Geometry: final body of the model. Coordinates: model frame, mm. Face numbers are marked on the shaded views. A direction names the side the tool comes from. Round coordinates to 2 decimals unless told otherwise and drop trailing zeros. Loops run counter-clockwise (first coordinate to the right, second up) from the corner with the lowest first, then second, coordinate; pieces in that order, holes last. Notation, with made-up numbers: (-4.75, -35) -> (50.25, -35) arc R36 cw to (50.25, 4) -> close; hole circle Ø5 at (-14.75, -34.5). An arc over 180 degrees is marked (long way). Answer in a Markdown table with one row per item.
```python
from build123d import *

# Parameters (mm, degrees)
SKETCH_W        = 83
SKETCH_H        = 20
PAD_DEPTH       = 3
SKETCH001_W     = 3
SKETCH001_H     = 20
PAD001_DEPTH    = 25
SKETCH002_W     = 30
SKETCH002_H     = 20
PAD002_DEPTH    = 50
POCKET_DEPTH    = 20.001
POCKET001_DEPTH = 53.001
SKETCH006_W     = 3
SKETCH006_H     = 20
PAD003_DEPTH    = 10
SKETCH007_W     = 20
SKETCH007_H     = 3
PAD004_DEPTH    = 5


with BuildPart() as part:
    # Sketch → Pad (new body)
    with BuildSketch(Plane.XY):
        Rectangle(SKETCH_W, SKETCH_H)
    extrude(amount=PAD_DEPTH)

    # Sketch001 → Pad001 (new body)
    with BuildSketch(Plane.XY.offset(3)):
        with Locations((-40, 0)):
            Rectangle(SKETCH001_W, SKETCH001_H)
    extrude(amount=PAD001_DEPTH)

    # Sketch002 → Pad002 (new body)
    with BuildSketch(Plane.XY.offset(3)):
        with Locations((14.5, 0)):
            Rectangle(SKETCH002_W, SKETCH002_H)
    extrude(amount=PAD002_DEPTH)

    # Sketch004 → Pocket (cut, through all)
    with BuildSketch(Plane.XZ.offset(10)):
        with BuildLine():
            Line((2.5, 53), (6.936769, 23.329896))
            ThreePointArc((6.936769, 23.329896), (11.333368, 13.220729), (20.195517, 6.664232))
            Line((20.195517, 6.664232), (29.5, 3))
            Line((63.265705, 66.309877), (29.5, 3))
            Line((2.5, 53), (63.265705, 66.309877))
        make_face()
    extrude(amount=-POCKET_DEPTH, mode=Mode.SUBTRACT)

    # Sketch005 → Pocket001 (cut, through all)
    with BuildSketch(Plane(origin=(0, 0, 0), x_dir=(1, 0, 0), z_dir=(0, 0, -1))):
        with BuildLine():
            ThreePointArc((-25.5, 7), (-32.5, 0), (-25.5, -7))
            Line((-25.5, -7), (29.5, -7))
            ThreePointArc((29.5, -7), (36.5, 0), (29.5, 7))
            Line((-25.5, 7), (29.5, 7))
        make_face()
    extrude(amount=-POCKET001_DEPTH, mode=Mode.SUBTRACT)

    # Sketch006 → Pad003 (new body)
    with BuildSketch(Plane(origin=(0, 0, 0), x_dir=(1, 0, 0), z_dir=(0, 0, -1))):
        with Locations((40, 0)):
            Rectangle(SKETCH006_W, SKETCH006_H)
    extrude(amount=PAD003_DEPTH)

    # Sketch007 → Pad004 (new body)
    with BuildSketch(Plane(origin=(38.5, 0, 0), x_dir=(0, -1, 0), z_dir=(-1, 0, 0))):
        with Locations((0, -8.5)):
            Rectangle(SKETCH007_W, SKETCH007_H)
    extrude(amount=PAD004_DEPTH)


solid = part.part
```
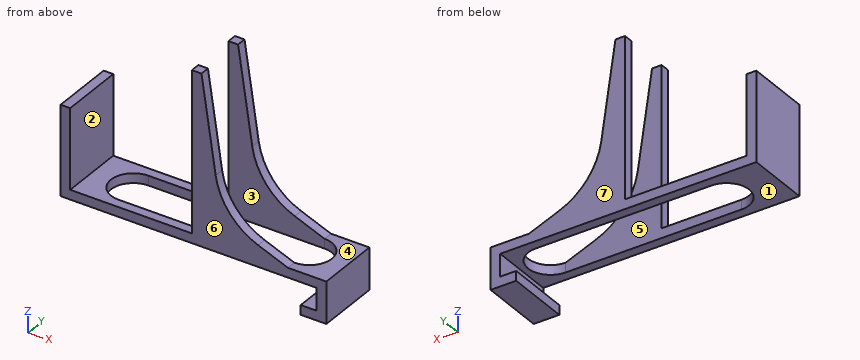
Item 1: Cut plane D-D (z = -5). Output: boundary loops of the cut face in (x, y), then the cut area to 3 significant figures.
Answer:
| item | result |
|---|---|
| outline | (38.5, -10) -> (41.5, -10) -> (41.5, 10) -> (38.5, 10) -> close |
| area | 60.0 mm² |
Item 2: Pin query (flat end, axial travel): pin 1 Ø12 at (x, y) = (19.5, -7) entering from +Z; pin 2 Ø3.5 at (x, y) = (-40.5, -4.5) entering from +Z; pin 3 Ø6 at (y, z) = (-1.5, 18.5) entering from +X. Return the tip coordinate at first contact, or that it passes through.
Answer:
| item | result |
|---|---|
| pin 1 | stops at z = 10.88 |
| pin 2 | stops at z = 28 |
| pin 3 | stops at x = -38.5 |
Item 3: Cut plane A-A (x = -23.5). Output: boundary loops of the cut face in (y, z), then the cut area to 3 significant figures.
Answer:
| item | result |
|---|---|
| outline | (-10, 0) -> (-7, 0) -> (-7, 3) -> (-10, 3) -> close; (7, 0) -> (10, 0) -> (10, 3) -> (7, 3) -> close |
| area | 18.0 mm² |
Item 4: Reachability of the marked faces 1, 2 and 3 from +Z, -Z, +X, -X, +Y, -Y: full face, straight path, thin tool, end or side. Return the list, or none.
Answer:
| item | result |
|---|---|
| face 1 | -X, +Y, -Y |
| face 2 | +Z, +Y, -Y |
| face 3 | +Z, -Z |
Item 5: Draft query along Y for the marked faces 4, 5, 6 and 7. Return one class per face: pulls with the +Y half, pulls with the -Y half, needs draft (parallel to the pull), parting line crosses it, or undercut.
Answer:
| item | result |
|---|---|
| face 4 | needs draft |
| face 5 | undercut |
| face 6 | pulls with the -Y half |
| face 7 | pulls with the +Y half |
Item 6: Cut plane B-B (y = -5.75). Output: boundary loops of the cut face in (x, z), then the cut area to 3 significant figures.
Answer:
| item | result |
|---|---|
| outline | (-41.5, 0) -> (-29.49, 0) -> (-29.49, 3) -> (-38.5, 3) -> (-38.5, 28) -> (-41.5, 28) -> close; (33.49, 0) -> (38.5, 0) -> (38.5, -7) -> (33.5, -7) -> (33.5, -10) -> (41.5, -10) -> (41.5, 3) -> (33.49, 3) -> close |
| area | 180 mm² |
Item 7: Cut plane C-C (y = 8.25). Output: boundary loops of the cut face in (x, z), then the cut area to 3 significant figures.
Answer:
| item | result |
|---|---|
| outline | (-41.5, 0) -> (38.5, 0) -> (38.5, -7) -> (33.5, -7) -> (33.5, -10) -> (41.5, -10) -> (41.5, 3) -> (29.5, 3) -> (20.2, 6.66) arc R21.3 cw to (6.94, 23.33) -> (2.5, 53) -> (-0.5, 53) -> (-0.5, 3) -> (-38.5, 3) -> (-38.5, 28) -> (-41.5, 28) -> close |
| area | 810 mm² |
Item 8: Line query: probe 1 along Y at (x, z) = (2, 36.5); probe 2 along Z at (x, y) = (34, 3.75); probe 3 along X at (y, z) = (4, 14.5). Output: solid intervals per line, ascending. Write a range as [from, to].
Answer:
| item | result |
|---|---|
| probe 1 | y = [-10, -7], [7, 10] |
| probe 2 | z = [-10, -7] |
| probe 3 | x = [-41.5, -38.5] |
